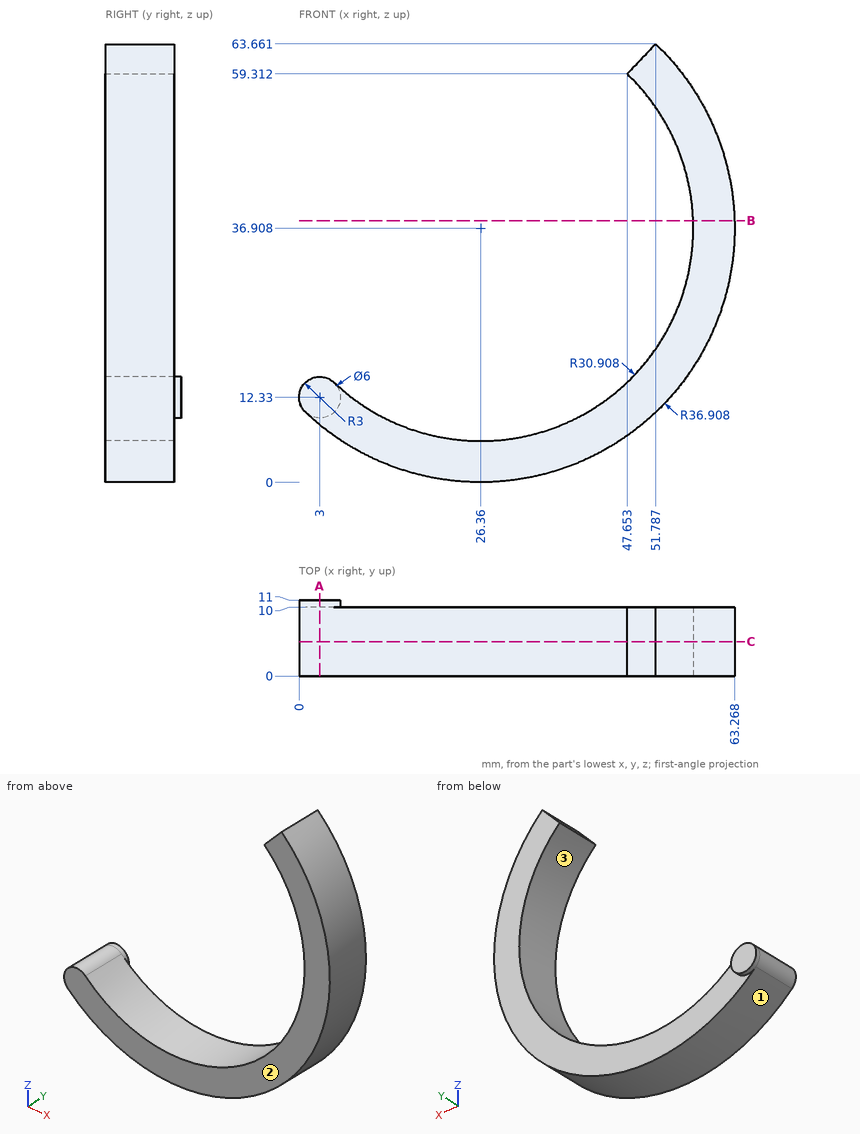
Geometry check sheet. Reference: drawing and pictorial views, mm from the part's lowest x, y, z. Coordinates: 2 decimals unless noted, no trailing zeros. Loops run counter-clockwise (first coordinate to the right, second up) from the corner with the lowest first, then second, coordinate; pieces in that order, holes last.
1) Gauge pin test, flat ends, axial feed: pin 1 (4 mm diameter, centred on x = 27, y = 8.5, fed in from -Z); pin 2 (2 mm diameter, centred on x = 43, y = 5.5, fed in from +Z); pin 3 (3 mm diameter, centred on x = 41, y = 3, fed in from -Z); pin 4 (8 mm diameter, centred on x = 28.5, z = 12, fed in from +Y) (3 decimals). Record the tip position at first contact, or that the pin passes through.
2) Sectioned sample at A-A (x = 3). Record the boundary of the cut face in (y, z).
3) Release check for a two-part mould opening along X. For the marked faces 1, 2 and 3 record: released by +X, released by -X, zero draft, split by the parting line, or undercut.
4) Sectioned sample at B-B (z = 38). Record the boundary of the cut face in (x, y).
5) Material ranges on probe 1 along Z at (x, y) = (54.5, 6.5) (1 decimal); probe 2 along Z at (x, y) = (27, 7.25) (1 decimal); probe 3 along Y at (x, z) = (59.5, 25), recorded low to high.
6) Sectioned sample at C-C (y = 5). Record the boundary of the cut face in (x, z) (1 decimal).
Check sheet entries:
1. pin 1: stops at z = 0
1. pin 2: stops at z = 11.53
1. pin 3: stops at z = 2.42
1. pin 4: passes through
2. outline: (0, 8.33) - (10, 8.33) - (10, 9.33) - (11, 9.33) - (11, 15.33) - (0, 15.33) - close
3. face 1: split by the parting line
3. face 2: zero draft
3. face 3: undercut
4. outline: (57.25, 0) - (63.25, 0) - (63.25, 10) - (57.25, 10) - close
5. probe 1: z = 13 to 24.1, 49.7 to 60.8
5. probe 2: z = 0 to 6
5. probe 3: y = 0 to 10
6. outline: (0.9, 10.2) arc R36.9 ccw to (51.8, 63.7) - (47.7, 59.3) arc R30.9 cw to (5.1, 14.5) arc R3 ccw to start
